Can you work these out from the model? Positions are in its coordinate system, mm. Give positions to 0.01 mm unless a question says otherwise; leave off trailing zeros. Loops run counter-clockwise (first coordinate to the right, second up) from the corner with the lowest first, then second, coordinate; pieces in that order, holes last. Notation, with made-up numbers: (82.5, 22) - (104.5, 22) arc R10 cw to (104.5, 38) - close; hole circle Ø9 at (-39, 86.25). An arc over 180 degrees is marked (long way). Answer as a JSON object with one key per item and string values.
```python
from build123d import *

# Parameters (mm, degrees)
SKETCH1_W           = 800
SKETCH1_H           = 800
BOSS_EXTRUDE1_DEPTH = 600
CUT_EXTRUDE1_DEPTH  = 801
CUT_EXTRUDE2_DEPTH  = 620.38214056
SKETCH4_R           = 1
BOSS_EXTRUDE2_DEPTH = 2


with BuildPart() as part:
    # Sketch1 → Boss-Extrude1 (new body)
    with BuildSketch(Plane.XY):
        with Locations((400, 400)):
            Rectangle(SKETCH1_W, SKETCH1_H)
    extrude(amount=BOSS_EXTRUDE1_DEPTH)

    # Sketch2 → Cut-Extrude1 (cut, through all)
    with BuildSketch(Plane(origin=(800, 0, 0), x_dir=(0, 0, -1), z_dir=(1, 0, 0))):
        Polygon((-600, 800), (-600, 401), (496.243490362, 800), align=None)
        Polygon((496.243490362, 0), (-600, 0), (-600, 399), align=None)
    extrude(amount=-CUT_EXTRUDE1_DEPTH, mode=Mode.SUBTRACT)

    # Sketch3 → Cut-Extrude2 (cut, through all)
    with BuildSketch(Plane.XZ):
        Polygon((401, 600), (800, -91.08827222), (800, 600), align=None)
        Polygon((0, 600), (0, -91.08827222), (399, 600), align=None)
    extrude(amount=-CUT_EXTRUDE2_DEPTH, mode=Mode.SUBTRACT)

    # Sketch4 → Boss-Extrude2 (add)
    with BuildSketch(Plane.XY.offset(600)):
        with Locations((400, 400)):
            Circle(SKETCH4_R)
    extrude(amount=BOSS_EXTRUDE2_DEPTH)


solid = part.part
```
1) I need wall thicknesses on L1, parallel to Y at x = 404.5, z = 489; L2, parallel to X at y = 446, z = 458; L3, parallel to Y at x = 425, z = 33.5. Which ranges of each line are inside material? Lowest first, please.
Check sheet entries:
{"L1": "358.6 to 441.4", "L2": "317.02 to 482.98", "L3": "192.81 to 607.19"}
2) Imagine slicing it at B-B on x = 322.5. Write out the boundary of the cut face in (y, z).
Check sheet entries:
{"outline": "(180.62, 0) - (619.38, 0) - (449.23, 467.5) - (350.77, 467.5) - close"}
3) Imagine slicing it at A-A on y = 537. Write out the boundary of the cut face in (x, z).
Check sheet entries:
{"outline": "(52.59, 0) - (747.41, 0) - (616.73, 226.34) - (183.27, 226.34) - close"}
4) I'm going to push flat-ended pins straight in: P1, Ø5, axis at x = 361, z = 293.5, coming from the +Y side; P2, Ø12, axis at x = 403, z = 181, coming from the -Y side; P3, Ø10, axis at y = 441, z = 66, coming from the -X side. Where does each tip first touch, or does it pass through?
Check sheet entries:
{"P1": "y = 513.47", "P2": "y = 244.31", "P3": "x = 87.81"}
